Part model, mm, in its own coordinate system. A direction names the side the tool comes from. Round coordinates to 2 decimals unless told otherwise and drop trailing zeros. Order: outer loops, then holes, each group sorted by start corner. A loop starts at its lowest first (then second) coordinate and runs counter-clockwise, first axis right, second up. Notation, with made-up numbers: M 82.5,83 L 98.5,83 A13 ccw 98.5,97 Z; hole C 19.5,45 d7. An arc over 180 degrees is marked long. One line per question, with ' | ' between items.
from build123d import *

# Parameters (mm, degrees)
SKETCH1_W           = 82
SKETCH1_H           = 73.66
BOSS_EXTRUDE1_DEPTH = 4
SKETCH2_W           = 4.88717895
SKETCH2_H           = 73.66
BOSS_EXTRUDE2_DEPTH = 100
SKETCH3_R           = 1.8125
CUT_EXTRUDE1_DEPTH  = 10
SKETCH4_W           = 24.37
SKETCH4_H           = 61.062715067
CUT_EXTRUDE2_DEPTH  = 10
SKETCH5_W           = 20.642645576
SKETCH5_H           = 101.129835632
SKETCH5_W_2         = 20.479187661
SKETCH5_H_2         = 100.180376076
CUT_EXTRUDE3_DEPTH  = 10


with BuildPart() as part:
    # Sketch1 → Boss-Extrude1 (new body)
    with BuildSketch(Plane(origin=(0, 0, 0), x_dir=(1, 0, 0), z_dir=(0, 1, 0))):
        with Locations((0.667646454, -2.157941762)):
            Rectangle(SKETCH1_W, SKETCH1_H)
    extrude(amount=BOSS_EXTRUDE1_DEPTH)

    # Sketch2 → Boss-Extrude2 (add)
    with BuildSketch(Plane(origin=(0, 4, 0), x_dir=(1, 0, 0), z_dir=(0, 1, 0))):
        with Locations((39.271911138, -2.157941762)):
            Rectangle(SKETCH2_W, SKETCH2_H)
    extrude(amount=BOSS_EXTRUDE2_DEPTH)

    # Sketch3 → Cut-Extrude1 (cut)
    with BuildSketch(Plane(origin=(0, 4, 0), x_dir=(1, 0, 0), z_dir=(0, 1, 0))):
        with Locations((-30.544050148, 9.782058238)):
            Circle(SKETCH3_R)
        with Locations((-30.544050148, -14.097941762)):
            Circle(SKETCH3_R)
    extrude(amount=-CUT_EXTRUDE1_DEPTH, mode=Mode.SUBTRACT)

    # Sketch4 → Cut-Extrude2 (cut)
    with BuildSketch(Plane(origin=(0, 4, 0), x_dir=(1, 0, 0), z_dir=(0, 1, 0))):
        with Locations((-13.885112628, -2.028636366)):
            Rectangle(SKETCH4_W, SKETCH4_H)
    extrude(amount=-CUT_EXTRUDE2_DEPTH, mode=Mode.SUBTRACT)

    # Sketch5 → Cut-Extrude3 (cut)
    with BuildSketch(Plane(origin=(41.715500613, 0, 0), x_dir=(0, 0, -1), z_dir=(1, 0, 0))):
        with Locations((15.687392669, 69.976580633)):
            Rectangle(SKETCH5_W, SKETCH5_H)
        with Locations((-20.375345347, 69.501850855)):
            Rectangle(SKETCH5_W_2, SKETCH5_H_2)
    extrude(amount=-CUT_EXTRUDE3_DEPTH, mode=Mode.SUBTRACT)


solid = part.part
1) Saw through at C-C (x = -14.5). List the corners of the cut face in (y, z), plus the area to 3 significant figures.
The answers:
outline: M 0,-34.67 L 4,-34.67 L 4,-28.5 L 0,-28.5 Z; M 0,32.56 L 4,32.56 L 4,38.99 L 0,38.99 Z | area: 50.4 mm²
2) Saw through at B-B (y = 87.5). List the corners of the cut face in (x, z).
The answers:
outline: M 36.83,-34.67 L 41.72,-34.67 L 41.72,-26.01 L 36.83,-26.01 Z; M 36.83,-5.37 L 41.72,-5.37 L 41.72,10.14 L 36.83,10.14 Z; M 36.83,30.61 L 41.72,30.61 L 41.72,38.99 L 36.83,38.99 Z
3) Which spindle directions (+Z, -Z, +X, -X, +Y, -Y) get a long thin tool onto all of the face, cutting with end or side? Do faces 1 (the face through (-26.07, 2, 2)), 2 (the face through (6, 4, 2)), 3 (the face through (41.716, 42, 3)), 4 (the face through (0, 0, 2)), 5 (the face through (39, 19.412, 21)). Say none if no direction does.
The answers:
face 1: +Y, -Y | face 2: +Z, -Z, -X, +Y | face 3: +Z, -Z, +X, +Y, -Y | face 4: +Z, -Z, +X, -X, -Y | face 5: +X, -X, +Y
4) Saw through at A-A (z = 25). List the corners of the cut face in (x, y).
The answers:
outline: M -40.33,0 L -26.07,0 L -26.07,4 L -40.33,4 Z; M -1.7,0 L 41.67,0 L 41.67,4 L 41.72,4 L 41.72,19.41 L 36.83,19.41 L 36.83,4 L -1.7,4 Z
5) Drop flat-ended pins along their axis: pin 1 (1.5 mm diameter, centred on x = 5, z = 10, fed in from +Y); pin 2 (1.2 mm diameter, centred on y = 1.5, z = -2.5, fed in from +X); pin 3 (2.5 mm diameter, centred on x = 39, z = -12, fed in from +Y). Give the stop position or say it passes through.
The answers:
pin 1: stops at y = 4 | pin 2: stops at x = 41.67 | pin 3: stops at y = 19.41
6) Saw through at D-D (z = -3). List the corners of the cut face in (x, y), plus the area to 3 significant figures.
The answers:
outline: M -40.33,0 L -26.07,0 L -26.07,4 L -40.33,4 Z; M -1.7,0 L 41.67,0 L 41.67,4 L 41.72,4 L 41.72,104 L 36.83,104 L 36.83,4 L -1.7,4 Z | area: 719 mm²
7) Probe line 1 (Y direction, x = -1, z = -15); line 2 (X direction, y = 35.5, z = -29). List the from-to ranges inside material, lowest first. Write a range as [from, to].
The answers:
line 1: y = [0, 4] | line 2: x = [36.83, 41.72]
